CAD build for the part. Positions are in the model's coordinates, mm. Face numbers are marked on the shaded views. A direction names the side the tool comes from. Give positions to 0.01 mm unless a question says otherwise; leave off trailing zeros. Order: outer loops, then holes, each group sorted by start corner. A loop starts at its lowest first (then second) coordinate and runs counter-clockwise, first axis right, second up. Notation, with made-up numbers: M 30,-26 L 56,-26 A27 ccw 56,-8 Z; hole C 70,-13.75 d2. An arc over 180 degrees is marked long. Put each result on its own line as item: value. Start each with the question number.
1) Tool access for the marked faces 1 and 2: list every direction of +Z, -Z, +X, -X, +Y, -Y with a clear straight run to the whole face (end or side of a thin tool).
2) Cut at C-C (y = 25.5). Write the cut outline in (x, z).
3) Drill centre lines: line 1 (Y direction, x = 59.55, z = 15); line 2 (X direction, y = 39, z = 22); line 3 (Z direction, x = 34.5, y = 27.5). Where is each one in solid material? Low to high. Write a range as [from, to].
4) Cut at D-D (z = 25). Write the cut outline in (x, y).
5) Cut at B-B (z = 15). Write the cut outline in (x, y), and give its area (3 significant figures).
6) Cut at A-A (y = 17). Write the cut outline in (x, z).
7) Two-plate mould, pull along X, no slides. Class the marked faces 3, 4 and 5: released by +X, released by -X, zero draft, split by the parting line, or undercut.
8) Pin check, flat tips, straight feed: pin 1 (4 mm diameter, centred on x = 18, z = 16, fed in from +Y); pin 2 (0.6 mm diameter, centred on y = 14.5, z = 1, fed in from -X); pin 3 (7 mm diameter, centred on y = 17, z = 15, fed in from +X). Stop position of each tip, or through.
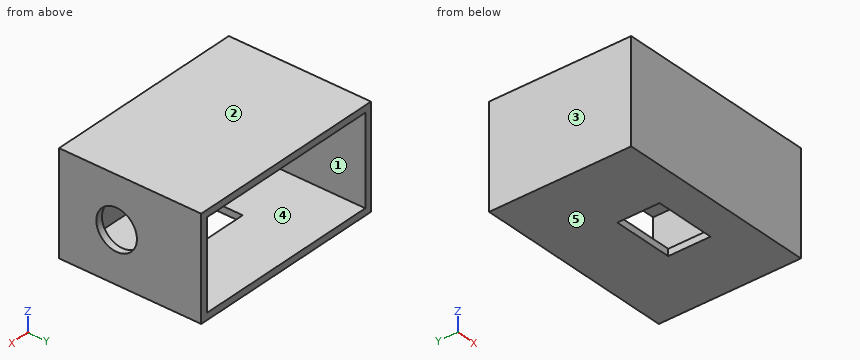
```python
from build123d import *

# Parameters (mm, degrees)
SKETCH1_W           = 60
SKETCH1_H           = 30
BOSS_EXTRUDE1_DEPTH = 2
SKETCH2_W           = 60
SKETCH2_H           = 2
BOSS_EXTRUDE2_DEPTH = 40
SKETCH3_W           = 60
SKETCH3_H           = 2
BOSS_EXTRUDE3_DEPTH = 40
SKETCH4_W           = 2
SKETCH4_H           = 26
BOSS_EXTRUDE4_DEPTH = 40
SKETCH5_W           = 2
SKETCH5_H           = 26
BOSS_EXTRUDE5_DEPTH = 40
CUT_EXTRUDE3_REACH  = 81.145
SKETCH7_R           = 6
CUT_EXTRUDE4_REACH  = 81.145
SKETCH8_W           = 18
SKETCH8_H           = 12.5


with BuildPart() as part:
    # Sketch1 → Boss-Extrude1 (new body)
    with BuildSketch(Plane(origin=(0, 0, 0), x_dir=(1, 0, 0), z_dir=(0, 1, 0))):
        with Locations((30, -15)):
            Rectangle(SKETCH1_W, SKETCH1_H)
    extrude(amount=BOSS_EXTRUDE1_DEPTH)

    # Sketch2 → Boss-Extrude2 (add)
    with BuildSketch(Plane(origin=(0, 2, 0), x_dir=(1, 0, 0), z_dir=(0, 1, 0))):
        with Locations((30, -1)):
            Rectangle(SKETCH2_W, SKETCH2_H)
    extrude(amount=BOSS_EXTRUDE2_DEPTH)

    # Sketch3 → Boss-Extrude3 (add)
    with BuildSketch(Plane(origin=(0, 2, 0), x_dir=(1, 0, 0), z_dir=(0, 1, 0))):
        with Locations((30, -29)):
            Rectangle(SKETCH3_W, SKETCH3_H)
    extrude(amount=BOSS_EXTRUDE3_DEPTH)

    # Sketch4 → Boss-Extrude4 (add)
    with BuildSketch(Plane(origin=(0, 2, 0), x_dir=(1, 0, 0), z_dir=(0, 1, 0))):
        with Locations((1, -15)):
            Rectangle(SKETCH4_W, SKETCH4_H)
    extrude(amount=BOSS_EXTRUDE4_DEPTH)

    # Sketch5 → Boss-Extrude5 (add)
    with BuildSketch(Plane(origin=(0, 2, 0), x_dir=(1, 0, 0), z_dir=(0, 1, 0))):
        with Locations((59, -15)):
            Rectangle(SKETCH5_W, SKETCH5_H)
    extrude(amount=BOSS_EXTRUDE5_DEPTH)

    # Sketch7 → Cut-Extrude3 (cut, up to next)
    with BuildSketch(Plane(origin=(60, 0, 0), x_dir=(0, 0, -1), z_dir=(1, 0, 0)), mode=Mode.PRIVATE) as cut_extrude3_sk1:
        with Locations((-15, 17)):
            Circle(SKETCH7_R)
    cut_extrude3_tool1 = extrude(cut_extrude3_sk1.sketch, amount=-CUT_EXTRUDE3_REACH, mode=Mode.PRIVATE) & part.part
    add(cut_extrude3_tool1.solids().sort_by_distance((60, 17, 15))[0], mode=Mode.SUBTRACT)

    # Sketch8 → Cut-Extrude4 (cut, up to next)
    with BuildSketch(Plane(origin=(0, 0, 0), x_dir=(-1, 0, 0), z_dir=(0, 0, -1)), mode=Mode.PRIVATE) as cut_extrude4_sk1:
        with Locations((-31, 16.25)):
            Rectangle(SKETCH8_W, SKETCH8_H)
    cut_extrude4_tool1 = extrude(cut_extrude4_sk1.sketch, amount=-CUT_EXTRUDE4_REACH, mode=Mode.PRIVATE) & part.part
    add(cut_extrude4_tool1.solids().sort_by_distance((31, 16.25, 0))[0], mode=Mode.SUBTRACT)


solid = part.part
```
Solution:
1. face 1: +Y
1. face 2: +Z, +X, -X, +Y, -Y
2. outline: M 0,0 L 60,0 L 60,30 L 0,30 Z; hole M 2,2 L 58,2 L 58,28 L 2,28 Z
3. line 1: [0, 11], [23, 42]
3. line 2: [0, 2], [58, 60]
3. line 3: [0, 2], [28, 30]
4. outline: M 0,0 L 60,0 L 60,42 L 58,42 L 58,2 L 2,2 L 2,42 L 0,42 Z
5. outline: M 0,0 L 60,0 L 60,11 L 58,11 L 58,2 L 2,2 L 2,42 L 0,42 Z; M 58,23 L 60,23 L 60,42 L 58,42 Z
5. area: 256 mm²
6. outline: M 0,0 L 22,0 L 22,2 L 2,2 L 2,28 L 58,28 L 58,21 L 60,21 L 60,30 L 0,30 Z; M 40,0 L 60,0 L 60,9 L 58,9 L 58,2 L 40,2 Z
7. face 3: released by -X
7. face 4: undercut
7. face 5: zero draft
8. pin 1: y = 2
8. pin 2: x = 0
8. pin 3: x = 2
